The model under review builds one solid part; all positions refer to its coordinate system, in mm. A direction names the side the tool comes from. Coordinates: 2 decimals unless noted, no trailing zeros. Write each loop counter-clockwise with the first axis right and the second up, starting at its lowest first coordinate (ties: lowest second). Pieces come first, ordered by that corner, then holes.
1) For P1, Ø6, axis at x = -9, z = 10.5, coming from the -Y side; P2, Ø3, axis at y = -8.5, z = -12.5, coming from the -X side; P3, Ø3, axis at x = -4, y = -10.5, coming from the +Z side; P4, Ø10, axis at y = 8.5, z = -21.5, coming from the -X side, all flat-tipped, find the tip position at first contact; note any pin that passes through.
2) Add section C-C, the plane y = 9. State the section outline as (x, z) points, then the cut area to 3 significant figures.
3) Mouldability with a two-part tool opening along X and no side actions: class faces 1 (the flat face through (-0.2, -6.5, 0)), 2 (the cylindrical face through (0.119, -0.677, -16.537)), 3 (the cylindrical face through (-14.985, -0.66, 12.325)) as released by +X, released by -X, zero draft, split by the parting line, or undercut.
4) Machinability: for faces 4 (the cylindrical face through (6, 0, -15)), 5 (the flat face through (0, 0, 3)), 6 (the flat face through (0, 4.5, -16)), which of the approach directions +Z, -Z, +X, -X, +Y, -Y give a long, thin tool a straight path to every point of the face, cutting with its end or side? Answer none if there is none.
5) Add section A-A, the plane y = 0. State the section outline as (x, z) points.
6) For line 1 (Z direction, x = 0, y = 2.75); line 2 (Y direction, x = 0, z = 11.75); line 3 (X direction, y = -0.25, z = -16), list the stretches that pass through material, from the lowest coordinate up.
7) Add section B-B, the plane x = 9.5. State the section outline as (y, z) points, then the cut area to 3 significant figures.
8) Add section D-D, the plane z = 6. State the section outline as (x, y) points, then the cut area to 3 significant figures.
Autodesk Inventor part; units mm, degrees
ref_plane "YZ Plane" through (0, 0, 0) normal (1, 0, 0) x (0, 1, 0)
ref_plane "XZ Plane" through (0, 0, 0) normal (0, 1, 0) x (-1, 0, 0)
ref_plane "XY Plane" through (0, 0, 0) normal (0, 0, 1) x (1, 0, 0)
sketch "Sketch1" plane through (0, 0, 0) normal (0, 0, 1) x (1, 0, 0)
  circle A0 centre (0, 0) radius 15
  dimension "d0" = 30
extrude "Extrusion1" add sketch "Sketch1" along normal blind 25
sketch "Sketch2" plane through (0, 0, 25) normal (0, 0, 1) x (1, 0, 0)
  circle A0 centre (0, 0) radius 14.5
  dimension "d3" = 29
extrude "Extrusion2" cut sketch "Sketch2" along normal blind 22
sketch "Sketch3" plane through (0, 0, 25) normal (0, 0, 1) x (1, 0, 0)
  circle A0 centre (0, 0) radius 14.5
  dimension "d6" = 29
extrude "Extrusion3" cut sketch "Sketch3" against normal blind 22
thread "Thread1"
sketch "Sketch4" plane through (0, 0, 0) normal (0, 0, -1) x (-1, 0, 0)
  circle A0 centre (0, 0) radius 6
  circle A1 centre (0, 0) radius 5
  dimension "d24" = 12
  dimension "d25" = 10
extrude "Extrusion4" add sketch "Sketch4" along normal blind 30 contours A0 | A1
sketch "Sketch5" plane through (0, 0, -30) normal (0, 0, -1) x (-1, 0, 0)
  point P0 (0, 0)
sketch "Sketch6" plane through (0, 0, 0) normal (0, 1, 0) x (-1, 0, 0)
  line L0 (-3.5, -20) -> (3.5, -20)
  line L1 (0, -20) -> (0, -16)
  circle A0 centre (0, -16) radius 0.55
  point P0 (0, 0)
  dimension "d14" = 4
  dimension "d15" = 1.1
extrude "Extrusion5" cut sketch "Sketch6" against normal blind 9 and the other way blind 4.5
sketch "Sketch7" plane through (0, 0, -30) normal (0, 0, -1) x (-1, 0, 0)
  point P0 (0, 0)
extrude "Extrusion6" [suppressed]
properties part number "CAPPER"
Geometry results:
1. P1: stops at y = -13.75
1. P2: passes through
1. P3: stops at z = 3
1. P4: stops at x = -4.87
2. outline: (-12, 0) - (12, 0) - (12, 25) - (11.37, 25) - (11.37, 3) - (-11.37, 3) - (-11.37, 25) - (-12, 25) - close
2. area: 99.8 mm2
3. face 1: zero draft
3. face 2: undercut
3. face 3: split by the parting line
4. face 4: -Z
4. face 5: +Z
4. face 6: -Y
5. outline: (-15, 0) - (-6, 0) - (-6, -30) - (6, -30) - (6, 0) - (15, 0) - (15, 25) - (14.5, 25) - (14.5, 3) - (-14.5, 3) - (-14.5, 25) - (-15, 25) - close; hole circle Ø1.1 at (0, -16)
6. line 1: z = -30 to -16.55, -15.45 to 3
6. line 2: y = -15 to -14.5, 14.5 to 15
6. line 3: x = -5.99 to -0.55, 0.55 to 5.99
7. outline: (-11.61, 0) - (11.61, 0) - (11.61, 25) - (10.95, 25) - (10.95, 3) - (-10.95, 3) - (-10.95, 25) - (-11.61, 25) - close
7. area: 98.4 mm2
8. outline: circle Ø30 at (0, 0); hole circle Ø29 at (0, 0)
8. area: 46.3 mm2
